Could you check a few things on this model? Use its own coordinates, in mm. Face numbers are marked on the shaded views. A direction names the side the tool comes from. Give positions to 0.01 mm unless a question says otherwise; leave off trailing zeros. Write each loop counter-clockwise with the first axis right and the second up, starting at its lowest first coordinate (ties: lowest second). Pieces come first, ordered by that corner, then holes. Notation, with made-up numbers: (67, -33) - (99, -33) arc R15 cw to (99, -27) - close; hole circle Ø3 at (40, -18.75). An arc over 180 degrees is marked (long way). Answer as a JSON object with one key per item and string values. Group by question number.
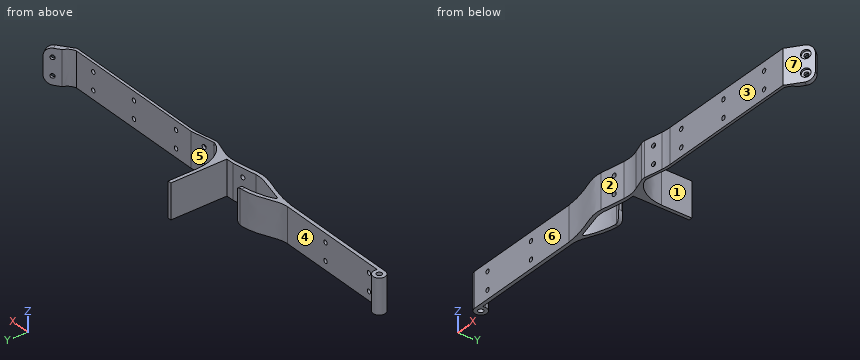
```python
from build123d import *

# Parameters (mm, degrees)
EXTRUDE_1_OUTLINE_R = 1.5
EXTRUDE_1_DEPTH     = 20
SKETCH_2_R          = 1.25
SKETCH_2_R_2        = 1.2
CUT_EXTRUDE_1_DEPTH = 20
SKETCH_3_R          = 1.25
CUT_EXTRUDE_2_DEPTH = 20
SKETCH_4_R          = 1.25
CUT_EXTRUDE_3_DEPTH = 20
SKETCH_9_R          = 1.25
CUT_EXTRUDE_5_DEPTH = 245.986373256
CUT_EXTRUDE_START   = -1.5
SKETCH_10_R         = 2.5
CUT_EXTRUDE_6_DEPTH = 10
FILLET_1_R          = 5
FILLET_2_R          = 5


# Read off the part's stored shape, not the designer's step: Бобышка-Вытянуть1
with BuildPart() as part:
    # Бобышка-Вытянуть1 outline → Бобышка-Вытянуть1 (new body)
    with BuildSketch(Plane(origin=(0, 0, 0), x_dir=(-1, 0, 0), z_dir=(0, 0, 1))):
        with BuildLine():
            add(Edge.make_bspline(
                [(142.011622395, 8.05757382), (150.943794363, 9.416584141), (156.347843346, 3.869799571), (171.865909279, 3.010474878)],
                knots=[0, 0, 0, 0, 1, 1, 1, 1], degree=3))
            Line((142.011622395, 8.05757382), (128.224313853, 5.626499332))
            ThreePointArc((128.224313853, 5.626499332), (123.301480263, 5.375276698), (118.466716866, 6.335727769))
            Line((118.466716866, 6.335727769), (111.443450657, 8.660414355))
            ThreePointArc((111.443450657, 8.660414355), (110.234759808, 8.900527123), (109.004051411, 8.837721464))
            Line((109.004051411, 8.837721464), (98.330959593, 6.955767409))
            ThreePointArc((98.330959593, 6.955767409), (95.736186546, 6.614159057), (93.121514264, 6.5))
            Line((93.121514264, 6.5), (10, 6.5))
            Line((10, 6.5), (-2.209609181, -2.534635535))
            Line((-2.209609181, -2.534635535), (-0.594520503, -4.762877579))
            Line((-0.594520503, -4.762877579), (6.692574577, 0.519001376))
            add(Edge.make_bspline(
                [(11.5, 5), (8.033807528, 3.95772064), (6.692574577, 0.519001376)],
                knots=[0, 0, 0, 1, 1, 1], degree=2))
            Line((11.5, 5), (95.877407164, 5))
            Line((95.877407164, 5), (109.629533412, 7.424870899))
            add(Edge.make_bspline(
                [(122, -11.220033081), (121.726076148, 0.257528082), (113.91616074, 7.041533795), (109.629533412, 7.424870899)],
                knots=[0, 0, 0, 0, 1, 1, 1, 1], degree=3))
            Line((122, -11.220033081), (122, -28.57498627))
            Line((122, -28.57498627), (123.999999999, -28.57498627))
            Line((123.999999999, -28.57498627), (123.999999999, 3.566059351))
            Line((123.999999999, 3.566059351), (128.571610209, 3.656883826))
            Line((128.571610209, 3.656883826), (142.358918751, 6.087958314))
            add(Edge.make_bspline(
                [(142.358918751, 6.087958314), (148.572133876, 6.8101534), (154.583213425, 3.766911307), (162.894761518, 2.067564733)],
                knots=[0, 0, 0, 0, 0.753728725, 0.753728725, 0.753728725, 0.753728725], degree=3))
            add(Edge.make_bspline(
                [(146.535286779, -4.560587457), (151.960770454, -4.769826895), (166.805940444, 0.965293), (162.894761518, 2.067564733)],
                knots=[0, 0, 0, 0, 1, 1, 1, 1], degree=3))
            add(Edge.make_bspline(
                [(146.535286779, -4.560587457), (144.68273182, -4.545804635), (143.745407166, -2.992935642), (142.704459303, -2.750002164)],
                knots=[0, 0, 0, 0, 1, 1, 1, 1], degree=3))
            Line((142.704459303, -2.750002164), (142.704459303, -4.750002164))
            add(Edge.make_bspline(
                [(146.535286779, -6.560587457), (143.834904881, -6.577431366), (142.704459303, -4.750002164)],
                knots=[0, 0, 0, 1, 1, 1], degree=2))
            add(Edge.make_bspline(
                [(171.865909279, 1.010474878), (163.771404707, 0.58774305), (159.000482555, -5.884509042), (146.535286779, -6.560587457)],
                knots=[0, 0, 0, 0, 1, 1, 1, 1], degree=3))
            Line((171.865909279, 1.010474878), (237.865909279, 1.010478432))
            Line((237.865909279, 1.010478432), (237.867088713, -0.489522958))
            ThreePointArc((237.867088713, -0.489522958), (243.841958753, -2.964395162), (241.367086549, 3.010474878))
            Line((241.367086549, 3.010474878), (171.865909279, 3.010474878))
        make_face()
        with Locations((241.367086549, -0.489522958)):
            Circle(EXTRUDE_1_OUTLINE_R, mode=Mode.SUBTRACT)
    extrude(amount=EXTRUDE_1_DEPTH)

    # Эскиз2 → Вырез-Вытянуть1 (cut)
    with BuildSketch(Plane.XZ.offset(6.5)):
        with Locations((-84.8, 15)):
            Circle(SKETCH_2_R)
        with Locations((-84.8, 5)):
            Circle(SKETCH_2_R)
        with Locations((-53.8, 15)):
            Circle(SKETCH_2_R)
        with Locations(Location((-231.865909279, 15, 0), (0, 0, 90))):
            Circle(SKETCH_2_R_2)
        with Locations(Location((-231.865909279, 5, 0), (0, 0, 90))):
            Circle(SKETCH_2_R_2)
        with Locations(Location((-199.865909279, 5, 0), (0, 0, 90))):
            Circle(SKETCH_2_R_2)
        with Locations(Location((-199.865909279, 15, 0), (0, 0, 90))):
            Circle(SKETCH_2_R_2)
        with Locations((-23.901835852, 15)):
            Circle(SKETCH_2_R)
        with Locations((-23.901835852, 5)):
            Circle(SKETCH_2_R)
        with Locations((-53.8, 5)):
            Circle(SKETCH_2_R)
    extrude(amount=-CUT_EXTRUDE_1_DEPTH, mode=Mode.SUBTRACT)

    # Эскиз3 → Вырез-Вытянуть2 (cut)
    with BuildSketch(Plane(origin=(-229.245460819, -28.516386222, 0), x_dir=(0.9848077530144649, 0.1736481776541319, 0), z_dir=(-0.17364817765413187, 0.9848077530144648, 0))):
        with Locations(Location((127.461195894, -15, 0), (0, 0, 180))):
            Circle(SKETCH_3_R)
        with Locations(Location((127.461195894, -5, 0), (0, 0, 180))):
            Circle(SKETCH_3_R)
    extrude(amount=-CUT_EXTRUDE_2_DEPTH, mode=Mode.SUBTRACT)

    # Эскиз4 → Вырез-Вытянуть3 (cut)
    with BuildSketch(Plane(origin=(-2.904248106, 16.470809483, 0), x_dir=(0.9848077530122088, 0.17364817766692647, 0), z_dir=(0.17364817766692645, -0.9848077530122087, 0))):
        with Locations((-133.123329763, 15)):
            Circle(SKETCH_4_R)
        with Locations((-133.123329763, 5)):
            Circle(SKETCH_4_R)
    extrude(amount=-CUT_EXTRUDE_3_DEPTH, mode=Mode.SUBTRACT)

    # Эскиз9 → Вырез-Вытянуть5 (cut, through all)
    with BuildSketch(Plane(origin=(-2.058456242, 2.839929973, 0), x_dir=(0.8096772311060745, 0.5868754394489519, 0), z_dir=(-0.5868754394489519, 0.8096772311060745, 0))):
        with Locations(Location((-1.223414413, -5, 0), (0, 0, 180))):
            Circle(SKETCH_9_R)
        with Locations(Location((-1.223414413, -15, 0), (0, 0, 180))):
            Circle(SKETCH_9_R)
    extrude(amount=-CUT_EXTRUDE_5_DEPTH, mode=Mode.SUBTRACT)

    # Эскиз10 → Вырез-Вытянуть6 (cut)
    with BuildSketch(Plane(origin=(-2.058456242, 2.839929973, 0), x_dir=(0.8096772311060745, 0.5868754394489519, 0), z_dir=(-0.5868754394489519, 0.8096772311060745, 0)).offset(CUT_EXTRUDE_START)):
        with Locations(Location((-1.223414413, -5, 0), (0, 0, 180))):
            Circle(SKETCH_10_R)
        with Locations(Location((-1.223414413, -15, 0), (0, 0, 180))):
            Circle(SKETCH_10_R)
    extrude(amount=-CUT_EXTRUDE_6_DEPTH, mode=Mode.SUBTRACT)

    # Скругление1
    fillet_1_edges = [part.edges().sort_by_distance(p)[0] for p in [
        (-142.704459303, 3.750002164, 0),
        (-142.704459303, 3.750002164, 20),
    ]]
    fillet(fillet_1_edges, radius=FILLET_1_R)

    # Скругление2
    fillet_2_edges = [part.edges().sort_by_distance(p)[0] for p in [
        (1.402064842, 3.648756557, 0),
        (1.402064842, 3.648756557, 20),
    ]]
    fillet(fillet_2_edges, radius=FILLET_2_R)


solid = part.part
```
(1) For the marked faces 1, 2, 3 and 4, which set-ups out of +Z, -Z, +X, -X, +Y, -Y let a thin tool reach every point of the face, with its end or its side?
(2) If we mould it in two halves opening along X, with no side actions, what happens to the marked faces 5, 6 and 7? For each: +X half, -X half, draft (parallel to the pull), parting line (faces both ways), or undercut.
(3) Will these pins go through, and if not, where does the flat tip stop? P1, Ø3, axis at x = -53.8, z = 15, coming from the +Y side; P2, Ø3, axis at y = 3, z = 10.5, coming from the -X side; P3, Ø1, axis at x = -128, z = 13, coming from the -Y side.
(4) I need wall thicknesses on L1, parallel to X at y = -1.95, z = 15; L2, parallel to Y at x = -41, z = 5.75; L3, parallel to Y at x = -220, z = 5.5. Which ranges of each line are inside material? Lowest first, please.
(5) I want a section at A-A, the plane y = 21. Please give me the cut outline in (x, z).
Entries:
{
 "1": {"face 1": "+Z, -Z, +X, +Y", "face 2": "+Z, -Z, -Y", "face 3": "+Z, -Z, +X, -Y", "face 4": "+Z, -Z, +Y"},
 "2": {"face 5": "undercut", "face 6": "draft", "face 7": "+X half"},
 "3": {"P1": "y = -5", "P2": "x = -244.72", "P3": "y = -5.68"},
 "4": {"L1": "-243.88 to -233.07, -230.67 to -201.07, -198.67 to -163.21, -124 to -117.56, -7.41 to -3.85", "L2": "-6.5 to -5", "L3": "-3.01 to -1.01"},
 "5": {"outline": "(-124, 0) - (-122, 0) - (-122, 20) - (-124, 20) - close"}
}
